from build123d import *

# Parameters (mm, degrees)
SKETCH2_OUTSIDE_W  = 41.142
SKETCH2_OUTSIDE_H  = 41.142
CUT_EXTRUDE1_DEPTH = 28.184554438
CUT_EXTRUDE3_DEPTH = 10


with BuildPart() as part:
    # Sketch1 → Revolve1 (revolve)
    with BuildSketch(Plane.XY, mode=Mode.PRIVATE) as revolve1_sk:
        Polygon((0, 3.9), (0, 5), (-1.35, 6.35), (-6.05, 6.35), (-7, 5.4), (-9, 5.4), (-9, 6.5), (-10.25, 6.5), (-10.25, 8.75), (-9, 8.75), (-9, 9), (-10.607695155, 15), (-15.392304845, 15), (-17, 9), (-17, 1.75), (-2.691303079, 1.75), (-1.45, 3.9), align=None)
    revolve(revolve1_sk.sketch.rotate(Axis((0, 0, 0), (-1, 0, 0)), 90), axis=Axis((0, 0, 0), (-1, 0, 0)))

    # Sketch2 outside → Cut-Extrude1 (cut, through all)
    with BuildSketch(Plane.ZY.offset(17)):
        Rectangle(SKETCH2_OUTSIDE_W, SKETCH2_OUTSIDE_H)
        Polygon((10.969655115, 0), (5.484827557, 9.5), (-5.484827557, 9.5), (-10.969655115, 0), (-5.484827557, -9.5), (5.484827557, -9.5), align=None, mode=Mode.SUBTRACT)
    extrude(amount=-CUT_EXTRUDE1_DEPTH, mode=Mode.SUBTRACT)

    # Sketch3 → Cut-Extrude3 (cut)
    with BuildSketch(Plane.XY.offset(4.95)):
        with BuildLine():
            Line((0, 1), (-7, 1))
            ThreePointArc((-7, 1), (-8, 0), (-7, -1))
            Line((-7, -1), (0, -1))
            Line((0, -1), (0, 0))
            Line((0, 0), (0, 1))
        make_face()
    extrude(amount=CUT_EXTRUDE3_DEPTH, mode=Mode.SUBTRACT)


solid = part.part
Input: part model. Units: mm. Frame: model coordinates. A direction names the side the tool comes from. Round coordinates to 2 decimals unless told otherwise and drop trailing zeros. Write each loop counter-clockwise with the first axis right and the second up, starting at its lowest first coordinate (ties: lowest second). Pieces come first, ordered by that corner, then holes.
1) Cut plane C-C (x = -3.75). Return the cut outline in (y, z).
2) Ray query, L1, parallel to Y at x = -9.5, z = 0; L2, parallel to X at y = 6.75, z = -0.5; L3, parallel to Y at x = -3.5, z = 0.75. Return the intervals inside material, ascending.
3) Draft query along Z for faces 6 (the conical face through (-2.61, -0.57, -1.8)), 7 (the cylindrical face through (-8.01, -1.62, -5.15)), 8 (the flat face through (-9, -4, -4)), 9 (the flat face through (-13.1, -4.8, 8.2)). Return one class per face: pulls with the +Z half, pulls with the -Z half, needs draft (parallel to the pull), parting line crosses it, or undercut.
4) Cut plane A-A (x = -12). Return the cut outline in (y, z), then the cut area to 3 significant figures.
5) Cut plane D-D (x = -2). Return the cut outline in (y, z), then the cut area to 3 significant figures.
6) Contact query for flat-ended pins moving along their axis: P1, Ø4, axis at y = 0, z = 0, coming from the +X side; P2, Ø3, axis at x = -10.5, y = 7.5, coming from the -Z side; P3, Ø1.5, axis at x = -9.5, y = 1, coming from the -Z side. Output: stop coordinate, or through.
7) Reachability of faces 1 (the cylindrical face through (-9.75, 1.55, -0.81)), 2 (the flat face through (-4, -1, 6)), 3 (the flat face through (-13, -9.5, 0)), 4 (the conical face through (-6.848, 0.232, -5.547)), 5 (the cylindrical face through (-0.71, -2.64, 2.87)) from +Z, -Z, +X, -X, +Y, -Y: full face, straight path, thin tool, end or side. Return the list, or none.
Geometry says:
1. outline: (-1, 4.95) - (-1, 6.27) arc R6.35 ccw (long way) to (1, 6.27) - (1, 4.95) - close; hole circle Ø3.5 at (0, 0)
2. L1: y = -9.5 to -8.75, -6.5 to -1.75, 1.75 to 6.5, 8.75 to 9.5
2. L2: x = -17 to -10.25
2. L3: y = -6.31 to -1.58, 1.58 to 6.31
3. face 6: undercut
3. face 7: parting line crosses it
3. face 8: needs draft
3. face 9: pulls with the +Z half
4. outline: (-9.5, -5.48) - (0, -10.97) - (9.5, -5.48) - (9.5, 5.48) - (0, 10.97) - (-9.5, 5.48) - close; hole circle Ø3.5 at (0, 0)
4. area: 303 mm2
5. outline: (-1, 4.95) - (-1, 6.27) arc R6.35 ccw (long way) to (1, 6.27) - (1, 4.95) - close; hole circle Ø5.89 at (0, 0)
5. area: 96.6 mm2
6. P1: stops at x = -2.55
6. P2: stops at z = -7.51
6. P3: stops at z = -10.83
7. face 1: +X, -X
7. face 2: +Z, +X
7. face 3: +Z, -Z, +X, -X, -Y
7. face 4: none
7. face 5: +X
